Can you work these out from the drawing? Everything is in mm from the part's minimum corner. A direction names the side the tool comes from. Round coordinates to 2 decimals unless told otherwise and drop trailing zeros. Loops run counter-clockwise (first coordinate to the right, second up) from the corner with the lowest first, then second, coordinate; pieces in that order, holes last. Notation, with made-up numbers: M 42,-32.75 L 88,-32.75 A28 ccw 88,-7.75 Z; hole C 63.5,-26 d6. An arc over 180 degrees is marked long. Answer in a Markdown table with one row per item.
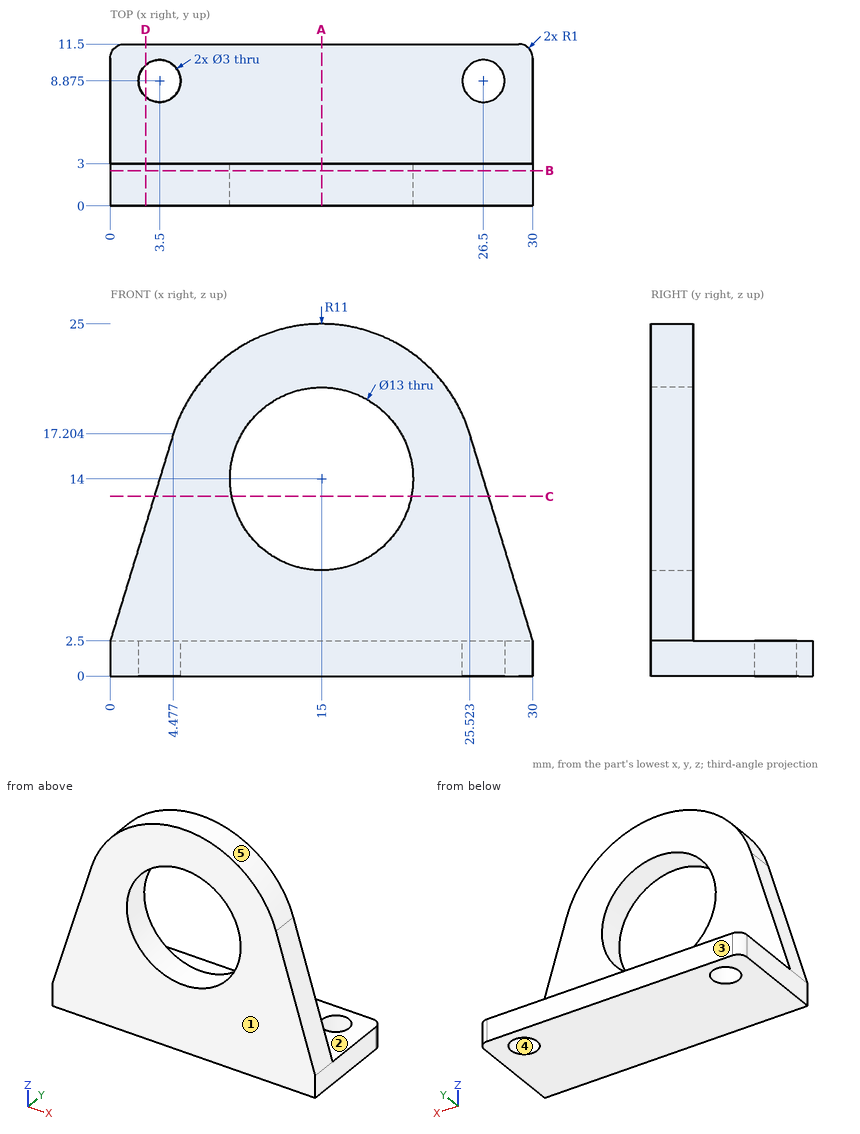
1) I want a section at A-A, the plane x = 15. Please give me the cut outline in (y, z).
Computed:
| item | result |
|---|---|
| outline | M 0,0 L 11.5,0 L 11.5,2.5 L 3,2.5 L 3,7.5 L 0,7.5 Z; M 0,20.5 L 3,20.5 L 3,25 L 0,25 Z |
2) I want a section at B-B, the plane y = 2.5. Please give me the cut outline in (x, z), plus the area to 3 significant figures.
Computed:
| item | result |
|---|---|
| outline | M 0,0 L 30,0 L 30,2.5 L 25.52,17.2 A11 ccw 4.48,17.2 L 0,2.5 Z; hole C 15,14 d13 |
| area | 438 mm² |
3) I want a section at C-C, the plane z = 12.75. Please give me the cut outline in (x, y), plus the area to 3 significant figures.
Computed:
| item | result |
|---|---|
| outline | M 3.12,0 L 8.62,0 L 8.62,3 L 3.12,3 Z; M 21.38,0 L 26.88,0 L 26.88,3 L 21.38,3 Z |
| area | 33.0 mm² |
4) Will these pins go through, and if not, where does the flat tip stop? P1, Ø2, axis at x = 4, z = 16.5, coming from the +Y side; P2, Ø4, axis at x = 16.5, y = 7, coming from the +Z side.
Computed:
| item | result |
|---|---|
| P1 | stops at y = 3 |
| P2 | stops at z = 2.5 |
5) I need wall thicknesses on line 1 (Y direction, x = 26.5, z = 0.7) (1 decimal); line 2 (Z direction, x = 5.5, y = 5.75); line 3 (Z direction, x = 20.25, y = 0.5) (1 decimal). Which ranges of each line are inside material? Lowest first, please.
Computed:
| item | result |
|---|---|
| line 1 | y = 0 to 7.4, 10.4 to 11.5 |
| line 2 | z = 0 to 2.5 |
| line 3 | z = 0 to 10.2, 17.8 to 23.7 |
6) Which directions (+Z, -Z, +X, -X, +Y, -Y) give clear straight access to the entire face, cutting with the end or side of a thin tool? Please do the marked faces 1 and 2.
Computed:
| item | result |
|---|---|
| face 1 | +Z, -Z, +X, -X, -Y |
| face 2 | +Z, +X, -X, +Y |
7) If we mould it in two halves opening along X, with no side actions, what happens to the marked faces 3, 4 and 5? For each: released by +X, released by -X, zero draft, split by the parting line, or undercut.
Computed:
| item | result |
|---|---|
| face 3 | zero draft |
| face 4 | undercut |
| face 5 | split by the parting line |
8) I want a section at D-D, the plane x = 2.5. Please give me the cut outline in (y, z), plus the area to 3 significant figures.
Computed:
| item | result |
|---|---|
| outline | M 0,0 L 7.76,0 L 7.76,2.5 L 3,2.5 L 3,10.71 L 0,10.71 Z; M 9.99,0 L 11.5,0 L 11.5,2.5 L 9.99,2.5 Z |
| area | 47.8 mm² |
